Here's how the part is built. I have some questions about the finished solid (model axes, mm). Coordinates: 2 decimals unless noted, no trailing zeros. Write each loop counter-clockwise with the first axis right and the second up, starting at its lowest first coordinate (ties: lowest second). Pieces come first, ordered by that corner, then holes. Notation, with made-up numbers: M 27,55.25 L 53,55.25 A20 ccw 53,70.25 Z; hole C -23,63.25 d3. An arc over 180 degrees is marked long. Use a Markdown table: item, result.
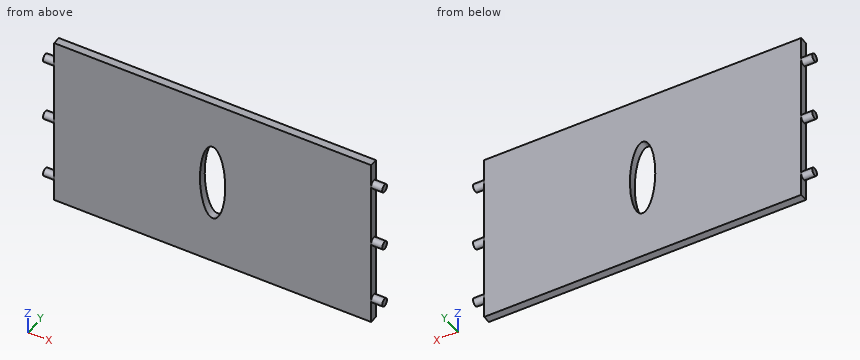
```python
from build123d import *

# Parameters (mm, degrees)
SKETCH1_W                = 200
SKETCH1_H                = 110
BOSS_EXTRUDE1_DEPTH      = 5
BOSS_EXTRUDE2_DEPTH      = 7
BOSS_EXTRUDE2_DEPTH_BACK = 207
SKETCH2_R                = 2.5
SKETCH3_RX               = 25
SKETCH3_RY               = 8
CUT_EXTRUDE1_DEPTH       = 10


with BuildPart() as part:
    # Sketch1 → Boss-Extrude1 (new body)
    with BuildSketch(Plane(origin=(0, 0, 0), x_dir=(1, 0, 0), z_dir=(0, 1, 0))):
        Rectangle(SKETCH1_W, SKETCH1_H)
    extrude(amount=BOSS_EXTRUDE1_DEPTH)

    # Sketch2 → Boss-Extrude2 (add, two sides: drawn at the far end of the back side and taken through both)
    with BuildSketch(Plane.ZY.offset(100).offset(-BOSS_EXTRUDE2_DEPTH_BACK)):
        with Locations((-40, 2.5)):
            Circle(SKETCH2_R)
        with Locations((0, 2.5)):
            Circle(SKETCH2_R)
        with Locations((40, 2.5)):
            Circle(SKETCH2_R)
    extrude(amount=BOSS_EXTRUDE2_DEPTH + BOSS_EXTRUDE2_DEPTH_BACK)

    # Sketch3 → Cut-Extrude1 (cut)
    with BuildSketch(Plane(origin=(0, 5, 0), x_dir=(1, 0, 0), z_dir=(0, 1, 0))):
        with Locations(Location((0, 0), (0, 0, 90))):
            Ellipse(SKETCH3_RX, SKETCH3_RY)
    extrude(amount=-CUT_EXTRUDE1_DEPTH, mode=Mode.SUBTRACT)


solid = part.part
```
1. I need wall thicknesses on probe 1 along X at (y, z) = (4.8, -35.5); probe 2 along X at (y, z) = (3.95, 13.5); probe 3 along X at (y, z) = (2.3, -12). Which ranges of each line are inside material? Lowest first, please.
Answers follow:
| item | result |
|---|---|
| probe 1 | x = -100 to 100 |
| probe 2 | x = -100 to -6.73, 6.73 to 100 |
| probe 3 | x = -100 to -7.02, 7.02 to 100 |
2. Suppose I cut it at A-A on z = -47. Write out the boundary of the cut face in (x, y).
Answers follow:
| item | result |
|---|---|
| outline | M -100,0 L 100,0 L 100,5 L -100,5 Z |
3. Will these pins go through, and if not, where does the flat tip stop? pin 1 Ø2.5 at (y, z) = (2, 45) entering from -X; pin 2 Ø2.5 at (y, z) = (3, -48) entering from +X.
Answers follow:
| item | result |
|---|---|
| pin 1 | stops at x = -100 |
| pin 2 | stops at x = 100 |
